from build123d import *

# Parameters (mm, degrees)
SKETCH_1_R      = 0.35
SKETCH_1_R_2    = 0.6
SKETCH_1_R_3    = 0.85
SKETCH_1_R_4    = 1.1
SKETCH_1_R_5    = 1.35
SKETCH_1_R_6    = 1.6
SKETCH_1_R_7    = 1.85
SKETCH_1_R_8    = 2.1
SKETCH_1_R_9    = 2.35
SKETCH_1_R_10   = 2.6
SKETCH_1_R_11   = 2.85
SKETCH_1_W      = 3
SKETCH_1_H      = 10
EXTRUDE_1_DEPTH = 3
FILLET_1_R      = 0.5
FILLET_2_R      = 1


with BuildPart() as part:
    # Эскиз1 → Бобышка-Вытянуть1 (new body)
    with BuildSketch(Plane.XY):
        Polygon((39, 19), (-39, 19), (-39, 16), (-52, 16), (-52, 5), (-52, -5), (-52, -19), (-49, -19), (-49, -22), (-46, -22), (-46, -19), (0, -19), (46, -19), (46, -22), (49, -22), (49, -19), (52, -19), (52, -5), (52, 5), (52, 16), (39, 16), align=None)
        with Locations((-37.65, -10.15)):
            Circle(SKETCH_1_R, mode=Mode.SUBTRACT)
        with Locations((-32.62, -10.15)):
            Circle(SKETCH_1_R_2, mode=Mode.SUBTRACT)
        with Locations((-27.09, -10.15)):
            Circle(SKETCH_1_R_3, mode=Mode.SUBTRACT)
        with Locations((-21.06, -10.15)):
            Circle(SKETCH_1_R_4, mode=Mode.SUBTRACT)
        with Locations((-14.53, -10.15)):
            Circle(SKETCH_1_R_5, mode=Mode.SUBTRACT)
        with Locations((-7.5, -10.15)):
            Circle(SKETCH_1_R_6, mode=Mode.SUBTRACT)
        with Locations((0.03, -10.15)):
            Circle(SKETCH_1_R_7, mode=Mode.SUBTRACT)
        with Locations((8.06, -10.15)):
            Circle(SKETCH_1_R_8, mode=Mode.SUBTRACT)
        with Locations((16.59, -10.15)):
            Circle(SKETCH_1_R_9, mode=Mode.SUBTRACT)
        with Locations((25.62, -10.15)):
            Circle(SKETCH_1_R_10, mode=Mode.SUBTRACT)
        with Locations((35.15, -10.15)):
            Circle(SKETCH_1_R_11, mode=Mode.SUBTRACT)
        with Locations((-37.65, 2.55)):
            Circle(SKETCH_1_R, mode=Mode.SUBTRACT)
        with Locations((-32.62, 2.55)):
            Circle(SKETCH_1_R_2, mode=Mode.SUBTRACT)
        with Locations((-27.09, 2.55)):
            Circle(SKETCH_1_R_3, mode=Mode.SUBTRACT)
        with Locations((-21.06, 2.55)):
            Circle(SKETCH_1_R_4, mode=Mode.SUBTRACT)
        with Locations((-14.53, 2.55)):
            Circle(SKETCH_1_R_5, mode=Mode.SUBTRACT)
        with Locations((-7.5, 2.55)):
            Circle(SKETCH_1_R_6, mode=Mode.SUBTRACT)
        with Locations((0.03, 2.55)):
            Circle(SKETCH_1_R_7, mode=Mode.SUBTRACT)
        with Locations((8.06, 2.55)):
            Circle(SKETCH_1_R_8, mode=Mode.SUBTRACT)
        with Locations((16.59, 2.55)):
            Circle(SKETCH_1_R_9, mode=Mode.SUBTRACT)
        with Locations((25.62, 2.55)):
            Circle(SKETCH_1_R_10, mode=Mode.SUBTRACT)
        with Locations((35.15, 2.55)):
            Circle(SKETCH_1_R_11, mode=Mode.SUBTRACT)
        with Locations((-53.5, 0)):
            Rectangle(SKETCH_1_W, SKETCH_1_H)
        with Locations((53.5, 0)):
            Rectangle(SKETCH_1_W, SKETCH_1_H)
    extrude(amount=EXTRUDE_1_DEPTH)

    # Скругление1
    fillet_1_edges = [part.edges().sort_by_distance(p)[0] for p in [
        (-55, -5, 1.5),
        (-55, 5, 1.5),
        (55, 5, 1.5),
        (55, -5, 1.5),
        (49, -22, 1.5),
        (46, -22, 1.5),
        (-46, -22, 1.5),
        (-49, -22, 1.5),
    ]]
    fillet(fillet_1_edges, radius=FILLET_1_R)

    # Скругление2
    fillet_2_edges = [part.edges().sort_by_distance(p)[0] for p in [
        (-52, -19, 1.5),
        (-52, 16, 1.5),
        (-39, 16, 1.5),
        (-39, 19, 1.5),
        (39, 19, 1.5),
        (39, 16, 1.5),
        (52, 16, 1.5),
        (52, -19, 1.5),
    ]]
    fillet(fillet_2_edges, radius=FILLET_2_R)


solid = part.part
Geometry: final body of the model. Coordinates: model frame, mm. A direction names the side the tool comes from. Coordinates: 2 decimals unless noted, no trailing zeros. Loops run counter-clockwise (first coordinate to the right, second up) from the corner with the lowest first, then second, coordinate; pieces in that order, holes last. Notation, with made-up numbers: (15, -33) - (26, -33) arc R15 ccw to (26, -10) - close; hole circle Ø6 at (82.5, 0.5). An arc over 180 degrees is marked (long way). Put each result on its own line as item: value. Start each with the question number.
Q1. Pull-direction query (X, two-part tool) for faces 1 (the cylindrical face through (-13.242, 2.956, 1.479)), 2 (the cylindrical face through (6.512, -8.731, 1.479)), 3 (the flat face through (-48, -22, 1)), 4 (the flat face through (-55, 0, 1)); classes: released by +X, released by -X, zero draft, split by the parting line, or undercut.
Q2. Cut plane D-D, the plane z = 2.1. Give the number of separate pieces and of enclosed holes in the cut face, and give its area (3 significant figures).
Q3. Cut plane B-B, the plane x = -14.53. Return loops of the section in (y, z), and give its area (3 significant figures).
Q4. Set-up query: faces 5 (the flat face through (52, 10, 1)), 6 (the flat face through (47, -22, 1)), 7 (the flat face through (-49, -20, 1)), 8 (the flat face through (-46, -20, 1)), 9 (the flat face through (-53, 5, 1)). Return all of +Z, -Z, +X, -X, +Y, -Y with unobstructed straight access to the full face (end or side cutting, diameter ignored); none if empty.
Q5. Cut plane A-A, the plane x = 25.62. Return loops of the section in (y, z), and give its area (3 significant figures).
Q6. Cut plane C-C, the plane y = -17. Return loops of the section in (x, z).
Q7. Line query: line 1 (Y direction, x = 0.03, z = 1.65); line 2 (Y direction, x = 8.06, z = 1.3); line 3 (X direction, y = -19.5, z = 1.55). Output: solid intervals per line, ascending.
Q8. Pin query (flat end, axial travel): pin 1 Ø1.2 at (y, z) = (-20.5, 2) entering from -X; pin 2 Ø1.5 at (y, z) = (10.5, 1) entering from -X; pin 3 Ø1.5 at (x, z) = (38, 2) entering from -Y. Return the tip coordinate at first contact, or that it passes through.
Filled sheet:
1. face 1: undercut
1. face 2: undercut
1. face 3: zero draft
1. face 4: released by -X
2. separate pieces: 1
2. enclosed holes: 22
2. area: 3,730 mm²
3. outline: (-19, 0) - (-11.5, 0) - (-11.5, 3) - (-19, 3) - close; (-8.8, 0) - (1.2, 0) - (1.2, 3) - (-8.8, 3) - close; (3.9, 0) - (19, 0) - (19, 3) - (3.9, 3) - close
3. area: 97.8 mm²
4. face 5: +Z, -Z, +X, +Y
4. face 6: +Z, -Z, +X, -X, -Y
4. face 7: +Z, -Z, -X, -Y
4. face 8: +Z, -Z, -Y
4. face 9: +Z, -Z, -X, +Y
5. outline: (-19, 0) - (-12.75, 0) - (-12.75, 3) - (-19, 3) - close; (-7.55, 0) - (-0.05, 0) - (-0.05, 3) - (-7.55, 3) - close; (5.15, 0) - (19, 0) - (19, 3) - (5.15, 3) - close
5. area: 82.8 mm²
6. outline: (-52, 0) - (52, 0) - (52, 3) - (-52, 3) - close
7. line 1: -19 to -12, -8.3 to 0.7, 4.4 to 19
7. line 2: -19 to -12.25, -8.05 to 0.45, 4.65 to 19
7. line 3: -49 to -46, 46 to 49
8. pin 1: x = -49
8. pin 2: x = -52
8. pin 3: y = -19
